```python
from build123d import *

# Parameters (mm, degrees)
SALIENTE_EXTRUIR1_DEPTH = 6
CROQUIS2_R              = 3.9
SALIENTE_EXTRUIR2_DEPTH = 6.8
CHAFL_N1_SIZE           = 1
REDONDEO1_R             = 0.6


with BuildPart() as part:
    # Croquis1 → Saliente-Extruir1 (new body)
    with BuildSketch(Plane(origin=(0, 0, 0), x_dir=(0, 1, 0), z_dir=(0, 0, 1))):
        Polygon((5.8, -2.402438662), (5.8, 2.402438662), (2.402438662, 5.8), (-2.402438662, 5.8), (-5.8, 2.402438662), (-5.8, -2.402438662), (-2.402438662, -5.8), (2.402438662, -5.8), align=None)
    extrude(amount=SALIENTE_EXTRUIR1_DEPTH)

    # Croquis2 → Saliente-Extruir2 (add)
    with BuildSketch(Plane.XY.offset(6)):
        Circle(CROQUIS2_R)
    extrude(amount=SALIENTE_EXTRUIR2_DEPTH)

    # Chaflán1
    chafl_n1_edges = [part.edges().sort_by_distance(p)[0] for p in [
        (-3.9, 0, 12.8),
    ]]
    chamfer(chafl_n1_edges, length=CHAFL_N1_SIZE)

    # Redondeo1
    redondeo1_edges = [part.edges().sort_by_distance(p)[0] for p in [
        (-3.9, 0, 6),
    ]]
    fillet(redondeo1_edges, radius=REDONDEO1_R)


solid = part.part
```
Check sheet for the modelled part. Datum: model origin and axes. Units: mm. A direction names the side the tool comes from. Give positions to 0.01 mm unless a question says otherwise; leave off trailing zeros. Write each loop counter-clockwise with the first axis right and the second up, starting at its lowest first coordinate (ties: lowest second). Pieces come first, ordered by that corner, then holes. Notation, with made-up numbers: (55, -0.75) - (94, -0.75) arc R8 cw to (94, 12.25) - close; hole circle Ø7 at (57, -12). An arc over 180 degrees is marked (long way). Answer as a JSON object with one key per item and string values. Group by question number.
1) Depth check by flat-ended pin: P1, Ø3, axis at x = 1, z = 11, coming from the -Y side; P2, Ø5, axis at y = 3.5, z = 11, coming from the -X side; P3, Ø5, axis at y = 2, z = 9, coming from the +X side. Enter the tip coordinate at first touch or a pass-through.
2) Access from +Z, -Z, +X, -X, +Y, -Y to the whole of each face (thin tool, end or side, straight path). Record for faces 1 (the face through (-2.87, 2.64, 9.16)), 2 (the face through (0, 5.8, 3)).
3) Sectioned sample at A-A (z = 5.5). Record the cut outline in (x, y), then the cut area to 3 significant figures.
4) Thickness scan on probe 1 along Z at (x, y) = (4.5, 0.5); probe 2 along Y at (x, z) = (5, 4.25); probe 3 along X at (y, z) = (4.5, 5.5). Record the ranges inside material, lowest first. Write a range as from..to.
5) Sectioned sample at D-D (z = 10.5). Record the cut outline in (x, y), then the cut area to 3 significant figures.
6) Sectioned sample at B-B (y = 0). Record the cut outline in (x, z).
Geometry results:
{
 "1": {"P1": "stops at y = -3.9", "P2": "stops at x = -3.77", "P3": "stops at x = 3.9"},
 "2": {"face 1": "+Z", "face 2": "+Z, -Z, +X, -X, +Y"},
 "3": {"outline": "(-5.8, -2.4) - (-2.4, -5.8) - (2.4, -5.8) - (5.8, -2.4) - (5.8, 2.4) - (2.4, 5.8) - (-2.4, 5.8) - (-5.8, 2.4) - close", "area": "111 mm^2"},
 "4": {"probe 1": "z = 0..6", "probe 2": "y = -3.2..3.2", "probe 3": "x = -3.7..3.7"},
 "5": {"outline": "circle Ø7.8 at (0, 0)", "area": "47.8 mm^2"},
 "6": {"outline": "(-5.8, 0) - (5.8, 0) - (5.8, 6) - (4.5, 6) arc R0.6 cw to (3.9, 6.6) - (3.9, 11.8) - (2.9, 12.8) - (-2.9, 12.8) - (-3.9, 11.8) - (-3.9, 6.6) arc R0.6 cw to (-4.5, 6) - (-5.8, 6) - close"}
}
